from build123d import *

# Parameters (mm, degrees)
SKETCH1_R           = 4.9
BOSS_EXTRUDE1_DEPTH = 0.35
SKETCH3_R           = 4
SKETCH3_R_2         = 3.5
BOSS_EXTRUDE2_DEPTH = 4.1
SKETCH4_R           = 4.9
SKETCH4_R_2         = 3.5
BOSS_EXTRUDE3_DEPTH = 0.35
CUT_EXTRUDE1_START  = -4.45
CUT_EXTRUDE1_DEPTH  = 4.45
SKETCH7_W           = 4.663594428
SKETCH7_H           = 2.003453707
CUT_EXTRUDE2_DEPTH  = 11.45
SKETCH8_R           = 1.6
CUT_EXTRUDE3_DEPTH  = 11.45
CUT_EXTRUDE5_DEPTH  = 11.45


with BuildPart() as part:
    # Sketch1 → Boss-Extrude1 (new body)
    with BuildSketch(Plane(origin=(0, 0, 0), x_dir=(1, 0, 0), z_dir=(0, 1, 0))):
        with Locations(Location((0, 0, 0), (0, 0, 270))):
            Circle(SKETCH1_R)
    extrude(amount=BOSS_EXTRUDE1_DEPTH)

    # Sketch3 → Boss-Extrude2 (add)
    with BuildSketch(Plane(origin=(0, 0.35, 0), x_dir=(1, 0, 0), z_dir=(0, 1, 0))):
        with Locations(Location((0, 0, 0), (0, 0, 270))):
            Circle(SKETCH3_R)
        with Locations(Location((0, 0, 0), (0, 0, 270))):
            Circle(SKETCH3_R_2, mode=Mode.SUBTRACT)
    extrude(amount=BOSS_EXTRUDE2_DEPTH)

    # Sketch4 → Boss-Extrude3 (add)
    with BuildSketch(Plane(origin=(0, 4.45, 0), x_dir=(1, 0, 0), z_dir=(0, 1, 0))):
        with Locations(Location((0, 0, 0), (0, 0, 270))):
            Circle(SKETCH4_R)
        with Locations(Location((0, 0, 0), (0, 0, 270))):
            Circle(SKETCH4_R_2, mode=Mode.SUBTRACT)
    extrude(amount=BOSS_EXTRUDE3_DEPTH)

    # Sketch5 → Cut-Extrude1 (cut)
    with BuildSketch(Plane(origin=(0, 4.8, 0), x_dir=(1, 0, 0), z_dir=(0, 1, 0)).offset(CUT_EXTRUDE1_START)):
        with BuildLine():
            Line((4.485667421, 1.972000961), (3.407070658, 0.801167605))
            ThreePointArc((3.407070658, 0.801167605), (3.476690042, 0.403269573), (3.5, 0))
            ThreePointArc((3.5, 0), (3.451272606, -0.581994331), (3.306447199, -1.147783482))
            Line((3.306447199, -1.147783482), (4.629026079, -1.606896874))
            ThreePointArc((4.629026079, -1.606896874), (4.831781648, -0.814792064), (4.9, 0))
            ThreePointArc((4.9, 0), (4.795298237, 1.007529066), (4.485667421, 1.972000961))
        make_face()
    extrude(amount=CUT_EXTRUDE1_DEPTH, mode=Mode.SUBTRACT)

    # Sketch7 → Cut-Extrude2 (cut)
    with BuildSketch(Plane.XY):
        with Locations((-0.477873166, 2.398273147)):
            Rectangle(SKETCH7_W, SKETCH7_H)
    extrude(amount=-CUT_EXTRUDE2_DEPTH, mode=Mode.SUBTRACT)

    # Sketch8 → Cut-Extrude3 (cut)
    with BuildSketch(Plane(origin=(0, 0.35, 0), x_dir=(1, 0, 0), z_dir=(0, 1, 0))):
        with Locations(Location((0, 0, 0), (0, 0, 270))):
            Circle(SKETCH8_R)
    extrude(amount=-CUT_EXTRUDE3_DEPTH, mode=Mode.SUBTRACT)

    # Sketch9 → Cut-Extrude5 (cut)
    with BuildSketch(Plane(origin=(0, 0, 0), x_dir=(0, 0, -1), z_dir=(1, 0, 0))):
        with BuildLine():
            ThreePointArc((0.192835364, 2.4), (0.075678076, 2.682842712), (-0.207164636, 2.8))
            Line((-0.207164636, 2.8), (-0.207164636, 2))
            ThreePointArc((-0.207164636, 2), (0.075678076, 2.117157288), (0.192835364, 2.4))
        make_face()
        with BuildLine():
            Line((-0.207164636, 2), (-0.207164636, 2.8))
            ThreePointArc((-0.207164636, 2.8), (-0.607164636, 2.4), (-0.207164636, 2))
        make_face()
    extrude(amount=-CUT_EXTRUDE5_DEPTH, mode=Mode.SUBTRACT)


solid = part.part
Could you check a few things on this model? Use its own coordinates, in mm. A direction names the side the tool comes from. Give positions to 0.01 mm unless a question says otherwise; leave off trailing zeros. Order: outer loops, then holes, each group sorted by start corner. A loop starts at its lowest first (then second) coordinate and runs counter-clockwise, first axis right, second up. Notation, with made-up numbers: (42.25, 2.5) -> (69.25, 2.5) arc R24 cw to (69.25, 16.5) -> close; hole circle Ø7 at (16, -4.5). An arc over 180 degrees is marked (long way). Answer in a Markdown table with one row per item. Add a question column.
Item 1: I'm going to push flat-ended pins straight in: P1, Ø0.6, axis at x = -0.5, z = -2.5, coming from the +Y side; P2, Ø1, axis at x = 0.5, y = 3.5, coming from the -Z side; P3, Ø0.5, axis at y = 3, z = -3, coming from the -X side. Where does each tip first touch, or does it pass through?
Item 2: Please list where these lines run through material, in increasing order: probe 1 along X at (y, z) = (0.25, 0); probe 2 along Y at (x, z) = (4, -2.5).
Item 3: Imagine slicing it at A-A (x = 0.75). List the corners of the cut face in (y, z) for me, and give its area (3 significant figures).
Item 4: Imagine slicing it at B-B (z = -4.5). List the corners of the cut face in (x, y) for me, and give its area (3 significant figures).
Item 5: For faces 1 (the flat face through (-2, 0, 0)), 2 (the cylindrical face through (-4.9, 4.62, 0.01)), 3 (the flat face through (3.52, 3.04, 1.22)), 4 (the cylindrical face through (-1.336, 2.544, 3.235)), 5 (the cylindrical face through (-3.354, 2.371, 2.18)), which set-ups out of +Z, -Z, +X, -X, +Y, -Y let a thin tool reach every point of the face, with its end or its side?
Item 6: Imagine slicing it at D-D (z = 0). List the corners of the cut face in (x, y) for me, and give its area (3 significant figures).
Item 7: Imagine slicing it at C-C (x = -2.5). List the corners of the cut face in (y, z) for me.
Item 8: We'd pull the mould along X, two halves only. Please class faces 6 (the flat face through (-4, 4.8, 0)), 7 (the flat face through (3.59, 3.04, -1)), 8 (the flat face through (2, 0.35, 0)), 9 (the cylindrical face through (1.472, 0.173, 4.674)): pulls with the +X half, pulls with the -X half, needs draft (parallel to the pull), parting line crosses it, or undercut.
Result:
| question | item | result |
|---|---|---|
| 1 | P1 | y = 0.35 |
| 1 | P2 | z = -4 |
| 1 | P3 | x = -2.9 |
| 2 | probe 1 | -4.9 to -1.6, 1.6 to 4.9 |
| 2 | probe 2 | 0 to 0.35, 4.45 to 4.8 |
| 3 | outline | (0, -4.84) -> (0.35, -4.84) -> (0.35, -3.93) -> (1.4, -3.93) -> (1.4, -3.42) -> (0.35, -3.42) -> (0.35, -1.41) -> (0, -1.41) -> close; (0, 1.41) -> (0.35, 1.41) -> (0.35, 3.42) -> (4.8, 3.42) -> (4.8, 4.84) -> (4.45, 4.84) -> (4.45, 3.93) -> (0.35, 3.93) -> (0.35, 4.84) -> (0, 4.84) -> close; (3.4, -3.93) -> (4.45, -3.93) -> (4.45, -4.84) -> (4.8, -4.84) -> (4.8, -3.42) -> (3.4, -3.42) -> close |
| 3 | area | 6.56 mm2 |
| 4 | outline | (-1.94, 0) -> (1.94, 0) -> (1.94, 0.35) -> (-1.94, 0.35) -> close; (-1.94, 4.45) -> (1.94, 4.45) -> (1.94, 4.8) -> (-1.94, 4.8) -> close |
| 4 | area | 2.71 mm2 |
| 5 | face 1 | +Z, -Z, +X, -X, -Y |
| 5 | face 2 | +Y, -Y |
| 5 | face 3 | +X, +Y |
| 5 | face 4 | +Y |
| 5 | face 5 | none |
| 6 | outline | (-4.9, 0) -> (-1.6, 0) -> (-1.6, 0.35) -> (-3.5, 0.35) -> (-3.5, 2.06) -> (-4, 2.06) -> (-4, 0.35) -> (-4.9, 0.35) -> close; (-4.9, 4.45) -> (-4, 4.45) -> (-4, 2.74) -> (-3.5, 2.74) -> (-3.5, 4.8) -> (-4.9, 4.8) -> close; (1.6, 0) -> (4.9, 0) -> (4.9, 0.35) -> (1.6, 0.35) -> close |
| 6 | area | 4.51 mm2 |
| 7 | outline | (0, -4.21) -> (0.35, -4.21) -> (0.35, -3.12) -> (1.4, -3.12) -> (1.4, -2.45) -> (0.35, -2.45) -> (0.35, 2.45) -> (4.8, 2.45) -> (4.8, 4.21) -> (4.45, 4.21) -> (4.45, 3.12) -> (0.35, 3.12) -> (0.35, 4.21) -> (0, 4.21) -> close; (3.4, -3.12) -> (4.45, -3.12) -> (4.45, -4.21) -> (4.8, -4.21) -> (4.8, -2.45) -> (3.4, -2.45) -> close |
| 8 | face 6 | needs draft |
| 8 | face 7 | pulls with the +X half |
| 8 | face 8 | undercut |
| 8 | face 9 | parting line crosses it |
